Work out the finished part from the listing and answer in its coordinate system (mm). Face numbers are marked on the shaded views. A direction names the side the tool comes from. Round coordinates to 2 decimals unless told otherwise and drop trailing zeros. Write each loop counter-clockwise with the first axis right and the second up, starting at its lowest first coordinate (ties: lowest second). Pieces come first, ordered by that corner, then holes. Notation, with made-up numbers: (82.25, 2) - (105.25, 2) arc R30 cw to (105.25, 30) - close; hole circle Ø2 at (-22, 83.25). An arc over 180 degrees is marked (long way). Write item = value, one per line. Start each with the question number.
from build123d import *

# Parameters (mm, degrees)
EXTRUDE_1_DEPTH          = 28.5
EXTRUDE_2_DEPTH          = 3
EXTRUDE_START            = 3
EXTRUDE_3_DEPTH          = 3
CUT_EXTRUDE_1_DEPTH      = 1
CUT_EXTRUDE_START        = -1
CUT_EXTRUDE_2_DEPTH      = 1
SKETCH_6_R               = 2
CUT_EXTRUDE_3_DEPTH      = 33
CUT_EXTRUDE_5_DEPTH      = 6
CUT_EXTRUDE_5_DEPTH_BACK = 6
SKETCH_7_R               = 1.6
CUT_EXTRUDE_6_DEPTH      = 6
CUT_EXTRUDE_6_DEPTH_BACK = 2
SKETCH_8_R               = 2.5
CUT_EXTRUDE_START_2      = 30.5
CUT_EXTRUDE_7_DEPTH      = 32.5


with BuildPart() as part:
    # 草图1 → 凸台-拉伸1 (new body)
    with BuildSketch(Plane.XY):
        with BuildLine():
            Line((-20.25, 0), (-20.25, 17.25))
            ThreePointArc((-20.25, 17.25), (-19.371320344, 19.371320344), (-17.25, 20.25))
            Line((-17.25, 20.25), (17.25, 20.25))
            ThreePointArc((17.25, 20.25), (19.371320344, 19.371320344), (20.25, 17.25))
            Line((20.25, 17.25), (20.25, 13))
            ThreePointArc((20.25, 13), (21.128679656, 10.878679656), (23.25, 10))
            Line((23.25, 10), (26.25, 10))
            Line((26.25, 10), (26.25, 15))
            Line((26.25, 15), (24.75, 15))
            ThreePointArc((24.75, 15), (22.628679656, 15.878679656), (21.75, 18))
            Line((21.75, 18), (21.75, 18.75))
            ThreePointArc((21.75, 18.75), (20.871320344, 20.871320344), (18.75, 21.75))
            Line((18.75, 21.75), (0, 21.75))
            Line((0, 21.75), (-18.75, 21.75))
            ThreePointArc((-18.75, 21.75), (-20.871320344, 20.871320344), (-21.75, 18.75))
            Line((-21.75, 18.75), (-21.75, 0))
            Line((-21.75, 0), (-20.25, 0))
        make_face()
    extrude(amount=EXTRUDE_1_DEPTH)

    # 草图2 → 凸台-拉伸2 (add)
    with BuildSketch(Plane.XY.offset(28.5)):
        with BuildLine():
            Line((-21.75, 0), (26.25, 0))
            Line((26.25, 0), (26.25, 15))
            Line((26.25, 15), (24.75, 15))
            ThreePointArc((24.75, 15), (22.628679656, 15.878679656), (21.75, 18))
            Line((21.75, 18), (21.75, 18.75))
            ThreePointArc((21.75, 18.75), (20.871320344, 20.871320344), (18.75, 21.75))
            Line((18.75, 21.75), (-18.75, 21.75))
            ThreePointArc((-18.75, 21.75), (-20.871320344, 20.871320344), (-21.75, 18.75))
            Line((-21.75, 18.75), (-21.75, 0))
        make_face()
    extrude(amount=EXTRUDE_2_DEPTH)

    # 草图3 → 凸台-拉伸3 (add)
    with BuildSketch(Plane(origin=(0, 0, 0), x_dir=(-1, 0, 0), z_dir=(0, 0, -1)).offset(EXTRUDE_START)):
        with BuildLine():
            Line((21.75, 0), (-26.25, 0))
            Line((-26.25, 0), (-26.25, 15))
            Line((-26.25, 15), (-24.75, 15))
            ThreePointArc((-24.75, 15), (-22.628679656, 15.878679656), (-21.75, 18))
            Line((-21.75, 18), (-21.75, 18.75))
            ThreePointArc((-21.75, 18.75), (-20.871320344, 20.871320344), (-18.75, 21.75))
            Line((-18.75, 21.75), (18.75, 21.75))
            ThreePointArc((18.75, 21.75), (20.871320344, 20.871320344), (21.75, 18.75))
            Line((21.75, 18.75), (21.75, 0))
        make_face()
    extrude(amount=-EXTRUDE_3_DEPTH)

    # 草图4 → 切除-拉伸1 (cut)
    with BuildSketch(Plane.XY.offset(31.5)):
        with BuildLine():
            Line((26.25, 13.25), (26.25, 0))
            Line((26.25, 0), (-20, 0))
            Line((-20, 0), (-20, 18))
            ThreePointArc((-20, 18), (-19.414213562, 19.414213562), (-18, 20))
            Line((-18, 20), (18, 20))
            ThreePointArc((18, 20), (19.414213562, 19.414213562), (20, 18))
            Line((20, 18), (20, 15.25))
            ThreePointArc((20, 15.25), (20.585786438, 13.835786438), (22, 13.25))
            Line((22, 13.25), (26.25, 13.25))
        make_face()
    extrude(amount=-CUT_EXTRUDE_1_DEPTH, mode=Mode.SUBTRACT)

    # 草图5 → 切除-拉伸2 (cut)
    with BuildSketch(Plane(origin=(0, 0, -3), x_dir=(-1, 0, 0), z_dir=(0, 0, -1)).offset(CUT_EXTRUDE_START)):
        with BuildLine():
            Line((0, 0), (20, 0))
            Line((20, 0), (20, 18))
            ThreePointArc((20, 18), (19.414213562, 19.414213562), (18, 20))
            Line((18, 20), (-18, 20))
            ThreePointArc((-18, 20), (-19.414213562, 19.414213562), (-20, 18))
            Line((-20, 18), (-20, 15.25))
            ThreePointArc((-20, 15.25), (-20.585786438, 13.835786438), (-22, 13.25))
            Line((-22, 13.25), (-26.25, 13.25))
            Line((-26.25, 13.25), (-26.25, 0))
            Line((-26.25, 0), (0, 0))
        make_face()
    extrude(amount=CUT_EXTRUDE_2_DEPTH, mode=Mode.SUBTRACT)

    # 草图6 → 切除-拉伸3 (cut)
    with BuildSketch(Plane.XY.offset(30.5)):
        with Locations(Location((-16, 16, 0), (0, 0, 180))):
            Circle(SKETCH_6_R)
        with Locations(Location((16, 16, 0), (0, 0, 180))):
            Circle(SKETCH_6_R)
        with BuildLine():
            Line((22.074047969, 0), (25.074047969, 0))
            ThreePointArc((25.074047969, 0), (23.574047969, 1.5), (22.074047969, 0))
        make_face()
        with BuildLine():
            Line((-11.543902494, 13.665222838), (-5.052849459, 7.174169802))
            ThreePointArc((-5.052849459, 7.174169802), (-4.48601855, 6.891164125), (-3.86288238, 7.005579185))
            ThreePointArc((-3.86288238, 7.005579185), (-3.061467459, 7.39103626), (-2.222222222, 7.685162874))
            ThreePointArc((-2.222222222, 7.685162874), (-1.700694746, 8.04488302), (-1.5, 8.645808233))
            Line((-1.5, 8.645808233), (-1.5, 17.82554347))
            ThreePointArc((-1.5, 17.82554347), (-1.843832677, 18.580158898), (-2.638888889, 18.815851441))
            ThreePointArc((-2.638888889, 18.815851441), (-7.270985215, 17.553711118), (-11.438839919, 15.170792376))
            ThreePointArc((-11.438839919, 15.170792376), (-11.834369763, 14.441942942), (-11.543902494, 13.665222838))
        make_face()
        with BuildLine():
            Line((1.5, 17.82554347), (1.5, 8.645808233))
            ThreePointArc((1.5, 8.645808233), (1.700694746, 8.04488302), (2.222222222, 7.685162874))
            ThreePointArc((2.222222222, 7.685162874), (3.061467459, 7.39103626), (3.86288238, 7.005579185))
            ThreePointArc((3.86288238, 7.005579185), (4.48601855, 6.891164125), (5.052849459, 7.174169802))
            Line((5.052849459, 7.174169802), (11.543902494, 13.665222838))
            ThreePointArc((11.543902494, 13.665222838), (11.834369763, 14.441942942), (11.438839919, 15.170792376))
            ThreePointArc((11.438839919, 15.170792376), (7.270985215, 17.553711118), (2.638888889, 18.815851441))
            ThreePointArc((2.638888889, 18.815851441), (1.843832677, 18.580158898), (1.5, 17.82554347))
        make_face()
        with BuildLine():
            Line((13.665222838, 11.543902494), (7.174169802, 5.052849459))
            ThreePointArc((7.174169802, 5.052849459), (6.891164125, 4.48601855), (7.005579185, 3.86288238))
            ThreePointArc((7.005579185, 3.86288238), (7.39103626, 3.061467459), (7.685162874, 2.222222222))
            ThreePointArc((7.685162874, 2.222222222), (8.04488302, 1.700694746), (8.645808233, 1.5))
            Line((8.645808233, 1.5), (17.82554347, 1.5))
            ThreePointArc((17.82554347, 1.5), (18.580158898, 1.843832677), (18.815851441, 2.638888889))
            ThreePointArc((18.815851441, 2.638888889), (17.553711118, 7.270985215), (15.170792376, 11.438839919))
            ThreePointArc((15.170792376, 11.438839919), (14.441942942, 11.834369763), (13.665222838, 11.543902494))
        make_face()
        with BuildLine():
            Line((-4, 0), (4, 0))
            ThreePointArc((4, 0), (0, 4), (-4, 0))
        make_face()
        with BuildLine():
            Line((-17.82554347, 1.5), (-8.645808233, 1.5))
            ThreePointArc((-8.645808233, 1.5), (-8.04488302, 1.700694746), (-7.685162874, 2.222222222))
            ThreePointArc((-7.685162874, 2.222222222), (-7.39103626, 3.061467459), (-7.005579185, 3.86288238))
            ThreePointArc((-7.005579185, 3.86288238), (-6.891164125, 4.48601855), (-7.174169802, 5.052849459))
            Line((-7.174169802, 5.052849459), (-13.665222838, 11.543902494))
            ThreePointArc((-13.665222838, 11.543902494), (-14.441942942, 11.834369763), (-15.170792376, 11.438839919))
            ThreePointArc((-15.170792376, 11.438839919), (-17.553711118, 7.270985215), (-18.815851441, 2.638888889))
            ThreePointArc((-18.815851441, 2.638888889), (-18.580158898, 1.843832677), (-17.82554347, 1.5))
        make_face()
    extrude(amount=-CUT_EXTRUDE_3_DEPTH, mode=Mode.SUBTRACT)

    # 草图7 → 切除-拉伸5 (cut, two sides: drawn at the far end of the back side and taken through both)
    with BuildSketch(Plane(origin=(0, 15, 0), x_dir=(1, 0, 0), z_dir=(0, 1, 0)).offset(-CUT_EXTRUDE_5_DEPTH_BACK)):
        with Locations(Location((23.25, -5.25, 0), (0, 0, 270))):
            Circle(SKETCH_7_R)
        with Locations(Location((23.25, -23.25, 0), (0, 0, 270))):
            Circle(SKETCH_7_R)
    extrude(amount=CUT_EXTRUDE_5_DEPTH + CUT_EXTRUDE_5_DEPTH_BACK, mode=Mode.SUBTRACT)

    # 草图8 → 切除-拉伸6 (cut, two sides: drawn at the far end of the back side and taken through both)
    with BuildSketch(Plane(origin=(0, 15, 0), x_dir=(1, 0, 0), z_dir=(0, 1, 0)).offset(-CUT_EXTRUDE_6_DEPTH_BACK)):
        with Locations(Location((23.25, -5.25, 0), (0, 0, 270))):
            Circle(SKETCH_8_R)
        with Locations(Location((23.25, -23.25, 0), (0, 0, 270))):
            Circle(SKETCH_8_R)
    extrude(amount=CUT_EXTRUDE_6_DEPTH + CUT_EXTRUDE_6_DEPTH_BACK, mode=Mode.SUBTRACT)

    # 草图9 → 切除-拉伸7 (cut)
    with BuildSketch(Plane.XY.offset(CUT_EXTRUDE_START_2)):
        with BuildLine():
            Line((-19, 0), (19, 0))
            ThreePointArc((19, 0), (3.706716118, 18.634920328), (-17.553711118, 7.270985215))
            ThreePointArc((-17.553711118, 7.270985215), (-18.634920328, 3.706716118), (-19, 0))
        make_face()
    extrude(amount=-CUT_EXTRUDE_7_DEPTH, mode=Mode.SUBTRACT)


solid = part.part
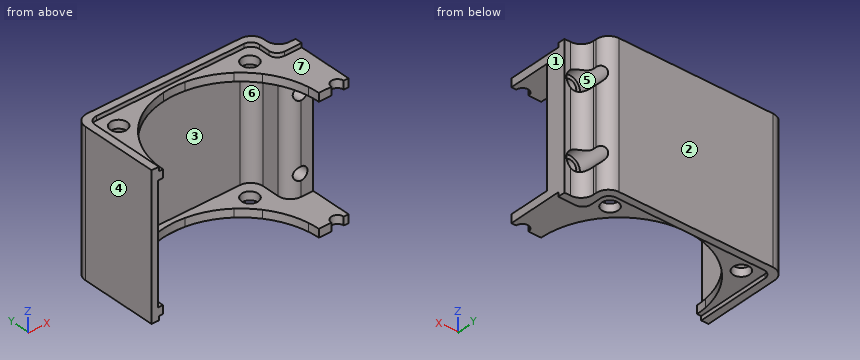
1. Consider line 1 (Z direction, x = 19, y = 12); line 2 (X direction, y = 16, z = -1.6); line 3 (Y direction, x = -12.5, z = 21.5). Determine where each line is inside the solid, lowest interval first.
2. For a pull along X with two mould halves and no side action, classify the marked faces 1, 2, 3 and 4 as released by +X, released by -X, zero draft, split by the parting line, or undercut.
3. Find section C-C on x = 16. Give the vertices of the cut face in (y, z), plus the area to 3 significant figures.
4. Which of the six approach directions +Z, -Z, +X, -X, +Y, -Y give full straight-line access (tool end or side, diameter ignored) to the marked faces 5, 6 and 7?
5. Find section A-A on z = 8.5. Give the vertices of the cut face in (x, y).
6. Find section D-D on z = 4.5. Give the vertices of the cut face in (x, y), plus the area to 3 significant figures.
7. Find section B-B on y = 8.25. Give the vertices of the cut face in (x, z).
8. Each of these flat-tipped pins is pushed along its axis until it touches: pin 1 (12 mm diameter, centred on x = 9.5, y = 4, fed in from -Z); pin 2 (2 mm diameter, centred on x = 12, z = 12, fed in from -Y); pin 3 (0.8 mm diameter, centred on y = 18, z = -1.5, fed in from +X); pin 4 (1.5 mm diameter, centred on y = 17.5, z = 18, fed in from +X). Where does it stop, or does it pass through?
Answer key:
q1.line_1 = -2 to 0, 28.5 to 30.5
q1.line_2 = -21.75 to -18, -14 to -10.25, 10.25 to 14, 18 to 22.51
q1.line_3 = 20.25 to 21.75
q2.face_1 = released by +X
q2.face_2 = zero draft
q2.face_3 = undercut
q2.face_4 = released by -X
q3.outline = (10.25, -2) - (14, -2) - (14, 0) - (10.25, 0) - close; (10.25, 28.5) - (14, 28.5) - (14, 30.5) - (10.25, 30.5) - close; (18, -2) - (20, -2) - (20, -3) - (21.75, -3) - (21.75, 31.5) - (20, 31.5) - (20, 30.5) - (18, 30.5) - (18, 28.5) - (20.25, 28.5) - (20.25, 0) - (18, 0) - close
q3.area = 76.3 mm²
q4.face_5 = +Y
q4.face_6 = -Y
q4.face_7 = +Z, -Y
q5.outline = (-21.75, 0) - (-20.25, 0) - (-20.25, 17.25) arc R3 cw to (-17.25, 20.25) - (17.25, 20.25) arc R3 cw to (20.25, 17.25) - (20.25, 13) arc R3 ccw to (23.25, 10) - (26.25, 10) - (26.25, 15) - (24.75, 15) arc R3 cw to (21.75, 18) - (21.75, 18.75) arc R3 ccw to (18.75, 21.75) - (-18.75, 21.75) arc R3 ccw to (-21.75, 18.75) - close
q6.outline = (-21.75, 0) - (-20.25, 0) - (-20.25, 17.25) arc R3 cw to (-17.25, 20.25) - (17.25, 20.25) arc R3 cw to (20.25, 17.25) - (20.25, 13) arc R3 ccw to (21.84, 10.35) - (21.84, 13) - (20.87, 13) - (20.87, 20.88) arc R3 ccw to (18.75, 21.75) - (-18.75, 21.75) arc R3 ccw to (-21.75, 18.75) - close; (24.66, 10) - (26.25, 10) - (26.25, 15) - (25.63, 15) - (25.63, 13) - (24.66, 13) - close
q6.area = 109 mm²
q7.outline = (-21.75, -3) - (-20, -3) - (-20, -2) - (-17.12, -2) - (-17.12, 0) - (-20.25, 0) - (-20.25, 28.5) - (-17.12, 28.5) - (-17.12, 30.5) - (-20, 30.5) - (-20, 31.5) - (-21.75, 31.5) - close; (17.12, -2) - (26.25, -2) - (26.25, 0) - (17.12, 0) - close; (17.12, 28.5) - (26.25, 28.5) - (26.25, 30.5) - (17.12, 30.5) - close
q8.pin_1 = through
q8.pin_2 = 20.25
q8.pin_3 = 21.78
q8.pin_4 = 22.02
